The listing builds one solid part. Answer for the finished solid, in the listing's coordinates (mm). A direction names the side the tool comes from. Round coordinates to 2 decimals unless told otherwise and drop trailing zeros. Write each loop counter-clockwise with the first axis right and the second up, starting at its lowest first coordinate (ties: lowest second). Pieces come first, ordered by that corner, then holes. Notation, with made-up numbers: (70.25, 58.25) - (87.25, 58.25) arc R33 ccw to (87.25, 87.25) - close; hole circle Ø5 at (28.5, 27). An arc over 180 degrees is marked (long way). Answer as CSV lines item,"result". Start each with the question number.
Item 1: A cutting plane is placed at B-B on z = 0.9. State how many separate pieces and enclosed holes the cut face has, and give its area (3 significant figures).
Item 2: A cutting plane is placed at C-C on y = 20. Determine the outline of the cut face in (x, z), and give its area (3 significant figures).
Item 3: Straight lines are drawn through the part: line 1 along X through (y, z) = (14.5, 1); line 2 along X through (y, z) = (15, 0.8); line 3 along Y through (x, z) = (50, 1.15). For each, find the intervals that lie inside material, in ascending order. Write a range as [from, to].
Item 4: A cutting plane is placed at A-A on x = 51. Determine the outline of the cut face in (y, z), and give its area (3 significant figures).
Item 5: Which of the six approach directions +Z, -Z, +X, -X, +Y, -Y give full straight-line access (tool end or side, diameter ignored) to faces 1 (the cylindrical face through (47.01, 12.36, 0.77)), 2 (the flat face through (51, 19, 1.57))?
Item 6: Flat-ended cylindrical pins translate along their axes: pin 1 (3.5 mm diameter, centred on x = 98.93, y = 26.48, fed in from +Z); pin 2 (5 mm diameter, centred on x = 98.93, y = 4, fed in from +Z); pin 3 (10 mm diameter, centred on x = 16.43, y = 18.9, fed in from -Z). Find the tip coordinate at first contact, or state that the pin passes through.
```python
from build123d import *

# Parameters (mm, degrees)
SKETCH1_W                                     = 102.87
SKETCH1_H                                     = 30.48
BOSS_EXTRUDE1_DEPTH                           = 1.57
FILLET1_R                                     = 3.935
CSK_FOR_6_FLAT_HEAD_MACHINE_SCREW1_AT_2_COUNT = 2
CSK_FOR_6_FLAT_HEAD_MACHINE_SCREW1_AT_2_PITCH = 22.479
CSK_FOR_6_FLAT_HEAD_MACHINE_SCREW1_AT_3_COUNT = 2
CSK_FOR_6_FLAT_HEAD_MACHINE_SCREW1_AT_3_PITCH = 94.996
CSK_FOR_6_FLAT_HEAD_MACHINE_SCREW1_AT_4_COUNT = 2
CSK_FOR_6_FLAT_HEAD_MACHINE_SCREW1_AT_4_PITCH = 97.619390784
DATA_SIDE_R                                   = 3.25
DATA_SIDE_R_2                                 = 2.5
CUT_EXTRUDE9_DEPTH                            = 1.57
MOVE_FACE4_BY                                 = 0.5
MOVE_FACE4_2_BY                               = 0.5
MOVE_FACE4_3_BY                               = 0.5
MOVE_FACE4_4_BY                               = 0.5
MOVE_FACE4_5_BY                               = 0.5
MOVE_FACE4_6_BY                               = 0.5
MOVE_FACE4_7_BY                               = 0.5
MOVE_FACE4_8_BY                               = 0.5
MOVE_FACE4_9_BY                               = 0.5
MOVE_FACE4_10_BY                              = 0.5


with BuildPart() as part:
    # Sketch1 → Boss-Extrude1 (new body)
    with BuildSketch(Plane.XY):
        with Locations((51.435, 15.24)):
            Rectangle(SKETCH1_W, SKETCH1_H)
    extrude(amount=BOSS_EXTRUDE1_DEPTH)

    # Fillet1
    fillet1_edges = [part.edges().sort_by_distance(p)[0] for p in [
        (0, 30.48, 0.785),
        (102.87, 30.48, 0.785),
        (102.87, 0, 0.785),
        (0, 0, 0.785),
    ]]
    fillet(fillet1_edges, radius=FILLET1_R)

    # Sketch4 → CSK for #6 Flat Head Machine Screw1 (revolve, cut)
    with BuildSketch(Plane(origin=(3.937, 26.4795, 1.57), x_dir=(0, -1, 0), z_dir=(1, 0, 0))):
        Polygon((0, 0), (0, 1.57), (2.0955, 1.57), (2.0955, 0.94962912), (2.921, 0), align=None)
    csk_for_6_flat_head_machine_screw1 = revolve(axis=Axis((3.937, 26.4795, 7.92), (0, 0, -1)), mode=Mode.SUBTRACT)

    # CSK for #6 Flat Head Machine Screw1 at 2: CSK for #6 Flat Head Machine Screw1 ×2
    with Locations(*[(0, -i * CSK_FOR_6_FLAT_HEAD_MACHINE_SCREW1_AT_2_PITCH, 0) for i in range(1, CSK_FOR_6_FLAT_HEAD_MACHINE_SCREW1_AT_2_COUNT)]):
        add(csk_for_6_flat_head_machine_screw1, mode=Mode.SUBTRACT)

    # CSK for #6 Flat Head Machine Screw1 at 3: CSK for #6 Flat Head Machine Screw1 ×2
    with Locations(*[(i * CSK_FOR_6_FLAT_HEAD_MACHINE_SCREW1_AT_3_PITCH, 0, 0) for i in range(1, CSK_FOR_6_FLAT_HEAD_MACHINE_SCREW1_AT_3_COUNT)]):
        add(csk_for_6_flat_head_machine_screw1, mode=Mode.SUBTRACT)

    # CSK for #6 Flat Head Machine Screw1 at 4: CSK for #6 Flat Head Machine Screw1 ×2
    with Locations(*[Vector(0.9731263352215668, -0.23027187344146696, 0) * (i * CSK_FOR_6_FLAT_HEAD_MACHINE_SCREW1_AT_4_PITCH) for i in range(1, CSK_FOR_6_FLAT_HEAD_MACHINE_SCREW1_AT_4_COUNT)]):
        add(csk_for_6_flat_head_machine_screw1, mode=Mode.SUBTRACT)

    # data side → Cut-Extrude9 (cut)
    with BuildSketch(Plane.XY):
        with Locations(Location((16.435, 18.8995, 0), (0, 0, 180))):
            Circle(DATA_SIDE_R)
        with Locations(Location((87.435, 14.8495, 0), (0, 0, 180))):
            Circle(DATA_SIDE_R_2)
        with BuildLine():
            Line((48.265, 15.7095), (54.605, 15.7095))
            ThreePointArc((54.605, 15.7095), (55.524238816, 15.328738816), (55.905, 14.4095))
            Line((55.905, 14.4095), (55.905, 13.6495))
            ThreePointArc((55.905, 13.6495), (55.524238816, 12.730261184), (54.605, 12.3495))
            Line((54.605, 12.3495), (48.265, 12.3495))
            ThreePointArc((48.265, 12.3495), (47.345761184, 12.730261184), (46.965, 13.6495))
            Line((46.965, 13.6495), (46.965, 14.4095))
            ThreePointArc((46.965, 14.4095), (47.345761184, 15.328738816), (48.265, 15.7095))
        make_face()
    extrude(amount=CUT_EXTRUDE9_DEPTH, mode=Mode.SUBTRACT)

    # Move Face4: a curved face moved inward by 0.5
    add(Solid.thicken(part.faces().sort_by_distance((89.935, 14.8495, 0.785))[0], -MOVE_FACE4_BY), mode=Mode.SUBTRACT)

    # Move Face4 2: a curved face moved inward by 0.5
    add(Solid.thicken(part.faces().sort_by_distance((19.685, 18.8995, 0.785))[0], -MOVE_FACE4_2_BY), mode=Mode.SUBTRACT)

    # Move Face4 3: a curved face moved inward by 0.5
    add(Solid.thicken(part.faces().sort_by_distance((55.524238816, 12.730261184, 0.785))[0], -MOVE_FACE4_3_BY), mode=Mode.SUBTRACT)

    # Move Face4 4: a curved face moved inward by 0.5
    add(Solid.thicken(part.faces().sort_by_distance((55.524238816, 15.328738816, 0.785))[0], -MOVE_FACE4_4_BY), mode=Mode.SUBTRACT)

    # Move Face4 5: a face moved inward by 0.5
    extrude(part.faces().sort_by_distance((55.905, 14.0295, 0.785))[0], amount=MOVE_FACE4_5_BY, dir=(1, 0, 0), mode=Mode.SUBTRACT)

    # Move Face4 6: a face moved inward by 0.5
    extrude(part.faces().sort_by_distance((51.435, 12.3495, 0.785))[0], amount=MOVE_FACE4_6_BY, dir=(0, -1, 0), mode=Mode.SUBTRACT)

    # Move Face4 7: a curved face moved inward by 0.5
    add(Solid.thicken(part.faces().sort_by_distance((47.345761184, 12.730261184, 0.785))[0], -MOVE_FACE4_7_BY), mode=Mode.SUBTRACT)

    # Move Face4 8: a face moved inward by 0.5
    extrude(part.faces().sort_by_distance((46.965, 14.0295, 0.785))[0], amount=MOVE_FACE4_8_BY, dir=(-1, 0, 0), mode=Mode.SUBTRACT)

    # Move Face4 9: a face moved inward by 0.5
    extrude(part.faces().sort_by_distance((51.435, 15.7095, 0.785))[0], amount=MOVE_FACE4_9_BY, dir=(0, 1, 0), mode=Mode.SUBTRACT)

    # Move Face4 10: a curved face moved inward by 0.5
    add(Solid.thicken(part.faces().sort_by_distance((47.345761184, 15.328738816, 0.785))[0], -MOVE_FACE4_10_BY), mode=Mode.SUBTRACT)


solid = part.part
```
Geometry says:
1,separate pieces,"1"
1,enclosed holes,"7"
1,area,"2,940 mm^2"
2,outline,"(0, 0) - (12.85, 0) - (12.85, 1.57) - (0, 1.57) - close; (20.02, 0) - (102.87, 0) - (102.87, 1.57) - (20.02, 1.57) - close"
2,area,"150 mm^2"
3,line 1,"x = [0, 46.47], [56.4, 84.46], [90.41, 102.87]"
3,line 2,"x = [0, 46.56], [56.31, 84.44], [90.43, 102.87]"
3,line 3,"y = [0, 11.85], [16.21, 30.48]"
4,outline,"(0, 0) - (11.85, 0) - (11.85, 1.57) - (0, 1.57) - close; (16.21, 0) - (30.48, 0) - (30.48, 1.57) - (16.21, 1.57) - close"
4,area,"41.0 mm^2"
5,face 1,"+Z, -Z"
5,face 2,"+Z, +X, -X, +Y, -Y"
6,pin 1,"passes through"
6,pin 2,"stops at z = 1.09"
6,pin 3,"stops at z = 0"
